Design review of the part built by this model. Coordinates are the model's own, in mm. A direction names the side the tool comes from. Coordinates: 2 decimals unless noted, no trailing zeros. Loops run counter-clockwise (first coordinate to the right, second up) from the corner with the lowest first, then second, coordinate; pieces in that order, holes last. Notation, with made-up numbers: M 80.25,19 L 102.25,19 A32 ccw 102.25,54 Z; hole C 43,16 d7. An arc over 180 degrees is marked long. Write item = value, one per line. Start each with the question number.
```python
from build123d import *

# Parameters (mm, degrees)
F1_DEPTH = 50
F2_W     = 25.7950418632
F2_H     = 50
F3_DEPTH = 9.8


with BuildPart() as f1:
    # F0 (on Front) → F1 (new body)
    with BuildSketch(Plane.XZ):
        with BuildLine():
            Line((28.7462828253, -6.7756745863), (26.6938590785, -11.5792195258))
            ThreePointArc((26.6938590785, -11.5792195258), (26.7363781025, -12.0511491494), (27.153647518, -12.2756745863))
            Line((27.153647518, -12.2756745863), (47.853647518, -12.2756745863))
            Line((47.853647518, -12.2756745863), (47.853647518, -11.4756745863))
            Line((47.853647518, -11.4756745863), (57.5962825562, -11.4756745863))
            Line((57.5962825562, -11.4756745863), (57.5962825562, 2.2953939865))
            Line((57.5962825562, 2.2953939865), (35.9046725562, 2.2953939865))
            Line((35.9046725562, 2.2953939865), (-33.5676551256, 8.3734350875))
            Line((-33.5676551256, 8.3734350875), (-81.6949312565, 21.2690998606))
            ThreePointArc((-81.6949312565, 21.2690998606), (-82.9196765939, 20.5619928104), (-82.2125695437, 19.337247473))
            Line((-82.2125695437, 19.337247473), (-33.9162782292, 6.3962952179))
            Line((-33.9162782292, 6.3962952179), (35.8173506372, 0.2953932255))
            Line((35.8173506372, 0.2953932255), (28.7462828253, -6.7756745863))
        make_face()
        Polygon((-33.9162782292, 6.3962952179), (28.7462828253, -6.7756745863), (35.8173506372, 0.2953932255), align=None)
    extrude(amount=F1_DEPTH)

    # F2 (on face) → F3 (cut)
    with BuildSketch(Plane(origin=(-0.1552477488, 0, -0.5793924863), x_dir=(0.9659258263, 0, -0.2588190451), z_dir=(0.2588190451, 0, 0.9659258263))):
        with BuildLine():
            Line((-84.4160920937, -50), (-59.5035807905, -50))
            ThreePointArc((-59.5035807905, -50), (-84.3714830361, -25), (-59.5035807905, 0))
            Line((-59.5035807905, 0), (-84.4160920937, 0))
            Line((-84.4160920937, 0), (-84.4160920937, -50))
        make_face()
        with Locations((-97.3136130253, -25)):
            Rectangle(F2_W, F2_H)
    extrude(amount=-F3_DEPTH, mode=Mode.SUBTRACT)

    # F4: F1 across face


with BuildPart() as f1_1:
    add(f1.part)
    add(f1.part.mirror(Plane(origin=(57.5962825562, -25, -4.5901402999), x_dir=(0, 1, 0), z_dir=(1, 0, 0))))


solid = f1_1.part
```
(1) To check wall thickness, follow L1, parallel to Z at x = 67, y = -33.5; L2, parallel to Z at x = 94, y = -10; L3, parallel to Z at x = 87, y = -43. State the ranges of each line that lie inside material, in increasing order.
(2) Take a section at B-B (y = -32). State the section outline as (x, z) points, plus the area to 3 significant figures.
(3) Insertion check: pin 1 (0.6 mm diameter, centred on y = -27.5, z = -12, fed in from -X); pin 2 (6 mm diameter, centred on x = 93.5, y = -5, fed in from +Z); pin 3 (3 mm diameter, centred on x = -25.5, y = -12, fed in from +Z). Each pin has a flat end and moves straight along its axis. Give the tip position at first contact, or say it passes through.
(4) Take a section at A-A (y = -4). State the section outline as (x, z) points, plus the area to 3 significant figures.
(5) Tool access review of faces 4 (the flat face through (58, -50, -2)), 5 (the cylindrical face through (197.094, -25.548, 20.304)), 6 (the flat face through (87.458, -24.65, -9.144)), 7 (the flat face through (57, -25, 2.295)), 8 (the flat face through (58, -25, -11.476)): name each direction out of +Z, -Z, +X, -X, +Y, -Y from which nothing blocks a thin tool from reaching the whole face with its end or side.
(6) Mouldability with a two-part tool opening along Z and no side actions: class faces 1 (the flat face through (173.57, -24.65, 12.95)), 2 (the flat face through (172.466, -24.65, 14.725)), 3 (the flat face through (27.734, -24.65, -9.144)) as +Z half, -Z half, draft (parallel to the pull), parting line (faces both ways), or undercut.
(7) Take a section at D-D (z = -0.5). State the section outline as (x, y) points.
(8) Take a section at C-C (x = -42.5). State the section outline as (y, z) points, plus the area to 3 significant figures.
Results list:
q1.L1 = -11.48 to 2.3
q1.L2 = -5.19 to 3.58
q1.L3 = -12.28 to -8.07, -6.66 to 2.97
q2.outline = M -81.2,19.07 L -33.92,6.4 L 28.75,-6.78 L 26.69,-11.58 A0.5 ccw 27.15,-12.28 L 47.85,-12.28 L 47.85,-11.48 L 67.34,-11.48 L 67.34,-12.28 L 88.04,-12.28 A0.5 ccw 88.5,-11.58 L 86.45,-6.78 L 149.11,6.4 L 196.4,19.07 L 195.88,21 L 148.76,8.37 L 79.29,2.3 L 35.9,2.3 L -33.57,8.37 L -80.69,21 Z
q2.area = 1,770 mm^2
q3.pin_1 = 26.65
q3.pin_2 = 3.8
q3.pin_3 = 7.8
q4.outline = M -71.12,16.37 L -33.92,6.4 L 28.75,-6.78 L 26.69,-11.58 A0.5 ccw 27.15,-12.28 L 47.85,-12.28 L 47.85,-11.48 L 67.34,-11.48 L 67.34,-12.28 L 88.04,-12.28 A0.5 ccw 88.5,-11.58 L 86.45,-6.78 L 149.11,6.4 L 186.32,16.37 L 185.8,18.3 L 148.76,8.37 L 79.29,2.3 L 35.9,2.3 L -33.57,8.37 L -70.61,18.3 Z
q4.area = 1,730 mm^2
q5.face_4 = +Z, -Z, +X, -X, -Y
q5.face_5 = +Z, +X
q5.face_6 = +X, +Y, -Y
q5.face_7 = +Z, +Y, -Y
q5.face_8 = -Z, +Y, -Y
q6.face_1 = -Z half
q6.face_2 = +Z half
q6.face_3 = undercut
q7.outline = M -1.11,-50 L 116.3,-50 L 116.3,0 L -1.11,0 Z
q8.outline = M -50,8.7 L 0,8.7 L 0,10.77 L -50,10.77 Z
q8.area = 104 mm^2
